The listing builds one solid part. Answer for the finished solid, in the listing's coordinates (mm). Face numbers are marked on the shaded views. A direction names the side the tool comes from. Coordinates: 2 decimals unless noted, no trailing zeros. Write each loop counter-clockwise with the first axis right and the second up, starting at its lowest first coordinate (ties: lowest second). Pieces come first, ordered by that corner, then holes.
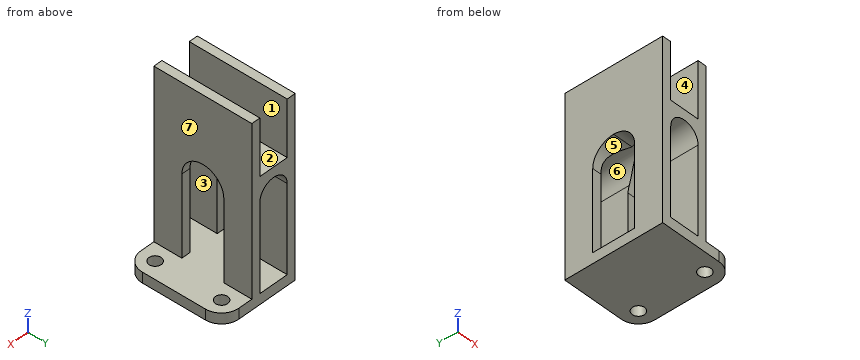
from build123d import *

# Parameters (mm, degrees)
F1_DEPTH     = 28
F2_R         = 1.75
F3_DEPTH     = 25
F4_W         = 12
F4_H         = 29
F5_DEPTH     = 25
F6_T4_DEPTH  = 28
F6_T10_DEPTH = 28
F6_T16_DEPTH = 28
F6_T23_DEPTH = 28
F6_T29_DEPTH = 28
F6_T35_DEPTH = 28
F6_T41_DEPTH = 28
F6_T47_DEPTH = 28
F6_T54_DEPTH = 28
F6_T60_DEPTH = 28
F7_R         = 5.99999
F8_R         = 5


# Not quite as in the source:
# - a fillet or chamfer that OpenCascade refuses, or shapes differently, is made with other operations: its cross-section is extruded or revolved along the edge and cut away or added
# - a fillet or chamfer is up to 0.001 mm smaller than in the source, because OpenCascade refuses the exact size


with BuildPart() as f1:
    # F0 (on Front) → F1 (new body)
    with BuildSketch(Plane.XZ):
        Polygon((-4.25, 25.5), (-6.75, 25.5), (-6.75, -22.5), (-6.75, -25.5), (-4.25, -25.5), (4.25, -25.5), (6.75, -25.5), (15.75, -25.5), (15.75, -22.5), (6.75, -22.5), (6.75, 25.5), (4.25, 25.5), (4.25, 9.5), (0, 9.5), (-4.25, 9.5), align=None)
        Polygon((4.25, -22.5), (-4.25, -22.5), (-4.25, 6.6576944664), (0, 6.6576944664), (4.25, 6.6576944664), align=None, mode=Mode.SUBTRACT)
    extrude(amount=F1_DEPTH)

    # F2 (on face) → F3 (cut)
    with BuildSketch(Plane(origin=(0, 0, -25.5), x_dir=(1, 0, 0), z_dir=(0, 0, -1))):
        with Locations((11.25, 23.5)):
            Circle(F2_R)
        with Locations((11.25, 4.5)):
            Circle(F2_R)
    extrude(amount=-F3_DEPTH, mode=Mode.SUBTRACT)

    # F4 (on face) → F5 (cut)
    with BuildSketch(Plane.YZ.offset(6.75)):
        with Locations((-14, -8)):
            Rectangle(F4_W, F4_H)
    extrude(amount=-F5_DEPTH, mode=Mode.SUBTRACT)

    # F6: fillet of radius 4.25 on 2 edges, made by hand


with BuildPart() as f6_tool2:
    # F6_s3 → F6_t4 (new body)
    with BuildSketch(Plane.XZ):
        with BuildLine():
            ThreePointArc((0, 6.6576944664), (3.00520382, 5.4128982865), (4.25, 2.4076944664))
            Line((4.25, 2.4076944664), (4.25, 6.6576944664))
            Line((4.25, 6.6576944664), (0, 6.6576944664))
        make_face()
    extrude(amount=F6_T4_DEPTH)

    split(bisect_by=Plane.XZ.offset(8), keep=Keep.BOTTOM)

    split(bisect_by=Plane.XY.offset(6.5), keep=Keep.TOP)


with BuildPart() as f1_1:
    add(f1.part)

    # F6_t1: union F6_tool2
    add(f6_tool2.part)


with BuildPart() as f6_tool8:
    # F6_s9 → F6_t10 (new body)
    with BuildSketch(Plane.XZ):
        with BuildLine():
            ThreePointArc((0, 6.6576944664), (3.00520382, 5.4128982865), (4.25, 2.4076944664))
            Line((4.25, 2.4076944664), (4.25, 6.6576944664))
            Line((4.25, 6.6576944664), (0, 6.6576944664))
        make_face()
    extrude(amount=F6_T10_DEPTH)

    split(bisect_by=Plane.XZ.offset(8), keep=Keep.BOTTOM)

    split(bisect_by=Plane.XY.offset(6.5), keep=Keep.BOTTOM)


with BuildPart() as f1_2:
    add(f1_1.part)

    # F6_t7: union F6_tool8
    add(f6_tool8.part)


with BuildPart() as f6_tool14:
    # F6_s15 → F6_t16 (new body)
    with BuildSketch(Plane.XZ):
        with BuildLine():
            ThreePointArc((0, 6.6576944664), (3.00520382, 5.4128982865), (4.25, 2.4076944664))
            Line((4.25, 2.4076944664), (4.25, 6.6576944664))
            Line((4.25, 6.6576944664), (0, 6.6576944664))
        make_face()
    extrude(amount=F6_T16_DEPTH)

    split(bisect_by=Plane.XZ.offset(8), keep=Keep.TOP)

    split(bisect_by=Plane.XY.offset(6.5), keep=Keep.TOP)

    split(bisect_by=Plane.XZ.offset(20), keep=Keep.BOTTOM)


with BuildPart() as f1_3:
    add(f1_2.part)

    # F6_t13: union F6_tool14
    add(f6_tool14.part)


with BuildPart() as f6_tool21:
    # F6_s22 → F6_t23 (new body)
    with BuildSketch(Plane.XZ):
        with BuildLine():
            ThreePointArc((0, 6.6576944664), (3.00520382, 5.4128982865), (4.25, 2.4076944664))
            Line((4.25, 2.4076944664), (4.25, 6.6576944664))
            Line((4.25, 6.6576944664), (0, 6.6576944664))
        make_face()
    extrude(amount=F6_T23_DEPTH)

    split(bisect_by=Plane.XY.offset(6.5), keep=Keep.TOP)

    split(bisect_by=Plane.XZ.offset(20), keep=Keep.TOP)


with BuildPart() as f1_4:
    add(f1_3.part)

    # F6_t20: union F6_tool21
    add(f6_tool21.part)


with BuildPart() as f6_tool27:
    # F6_s28 → F6_t29 (new body)
    with BuildSketch(Plane.XZ):
        with BuildLine():
            ThreePointArc((0, 6.6576944664), (3.00520382, 5.4128982865), (4.25, 2.4076944664))
            Line((4.25, 2.4076944664), (4.25, 6.6576944664))
            Line((4.25, 6.6576944664), (0, 6.6576944664))
        make_face()
    extrude(amount=F6_T29_DEPTH)

    split(bisect_by=Plane.XY.offset(6.5), keep=Keep.BOTTOM)

    split(bisect_by=Plane.XZ.offset(20), keep=Keep.TOP)


with BuildPart() as f1_5:
    add(f1_4.part)

    # F6_t26: union F6_tool27
    add(f6_tool27.part)


with BuildPart() as f6_tool33:
    # F6_s34 → F6_t35 (new body)
    with BuildSketch(Plane.XZ):
        with BuildLine():
            ThreePointArc((-4.25, 2.4076944664), (-3.00520382, 5.4128982865), (0, 6.6576944664))
            Line((0, 6.6576944664), (-4.25, 6.6576944664))
            Line((-4.25, 6.6576944664), (-4.25, 2.4076944664))
        make_face()
    extrude(amount=F6_T35_DEPTH)

    split(bisect_by=Plane.XZ.offset(8), keep=Keep.BOTTOM)

    split(bisect_by=Plane.XY.offset(6.5), keep=Keep.BOTTOM)


with BuildPart() as f1_6:
    add(f1_5.part)

    # F6_t32: union F6_tool33
    add(f6_tool33.part)


with BuildPart() as f6_tool39:
    # F6_s40 → F6_t41 (new body)
    with BuildSketch(Plane.XZ):
        with BuildLine():
            ThreePointArc((-4.25, 2.4076944664), (-3.00520382, 5.4128982865), (0, 6.6576944664))
            Line((0, 6.6576944664), (-4.25, 6.6576944664))
            Line((-4.25, 6.6576944664), (-4.25, 2.4076944664))
        make_face()
    extrude(amount=F6_T41_DEPTH)

    split(bisect_by=Plane.XZ.offset(8), keep=Keep.BOTTOM)

    split(bisect_by=Plane.XY.offset(6.5), keep=Keep.TOP)


with BuildPart() as f1_7:
    add(f1_6.part)

    # F6_t38: union F6_tool39
    add(f6_tool39.part)


with BuildPart() as f6_tool45:
    # F6_s46 → F6_t47 (new body)
    with BuildSketch(Plane.XZ):
        with BuildLine():
            ThreePointArc((-4.25, 2.4076944664), (-3.00520382, 5.4128982865), (0, 6.6576944664))
            Line((0, 6.6576944664), (-4.25, 6.6576944664))
            Line((-4.25, 6.6576944664), (-4.25, 2.4076944664))
        make_face()
    extrude(amount=F6_T47_DEPTH)

    split(bisect_by=Plane.XZ.offset(20), keep=Keep.BOTTOM)

    split(bisect_by=Plane.XZ.offset(8), keep=Keep.TOP)

    split(bisect_by=Plane.XY.offset(6.5), keep=Keep.TOP)


with BuildPart() as f1_8:
    add(f1_7.part)

    # F6_t44: union F6_tool45
    add(f6_tool45.part)


with BuildPart() as f6_tool52:
    # F6_s53 → F6_t54 (new body)
    with BuildSketch(Plane.XZ):
        with BuildLine():
            ThreePointArc((-4.25, 2.4076944664), (-3.00520382, 5.4128982865), (0, 6.6576944664))
            Line((0, 6.6576944664), (-4.25, 6.6576944664))
            Line((-4.25, 6.6576944664), (-4.25, 2.4076944664))
        make_face()
    extrude(amount=F6_T54_DEPTH)

    split(bisect_by=Plane.XZ.offset(20), keep=Keep.TOP)

    split(bisect_by=Plane.XY.offset(6.5), keep=Keep.BOTTOM)


with BuildPart() as f1_9:
    add(f1_8.part)

    # F6_t51: union F6_tool52
    add(f6_tool52.part)


with BuildPart() as f6_tool58:
    # F6_s59 → F6_t60 (new body)
    with BuildSketch(Plane.XZ):
        with BuildLine():
            ThreePointArc((-4.25, 2.4076944664), (-3.00520382, 5.4128982865), (0, 6.6576944664))
            Line((0, 6.6576944664), (-4.25, 6.6576944664))
            Line((-4.25, 6.6576944664), (-4.25, 2.4076944664))
        make_face()
    extrude(amount=F6_T60_DEPTH)

    split(bisect_by=Plane.XZ.offset(20), keep=Keep.TOP)

    split(bisect_by=Plane.XY.offset(6.5), keep=Keep.TOP)


with BuildPart() as f1_10:
    add(f1_9.part)

    # F6_t57: union F6_tool58
    add(f6_tool58.part)

    # F7 (radius 6 in the source; OpenCascade refuses exactly that, so slightly less here)
    f7_edges = [f1_10.edges().sort_by_distance(p)[0] for p in [
        (3.948484, -20, 6.5),
        (-3.948484, -20, 6.5),
        (-3.948484, -8, 6.5),
        (3.948484, -8, 6.5),
    ]]
    fillet(f7_edges, radius=F7_R)

    # F8
    f8_edges = [f1_10.edges().sort_by_distance(p)[0] for p in [
        (15.75, 0, -24),
        (15.75, -28, -24),
    ]]
    fillet(f8_edges, radius=F8_R)


solid = f1_10.part
Q1. Determine the mould class of the marked faces 1, 2 and 3 for opening direction Z: released by +Z, released by -Z, zero draft, split by the parting line, or undercut.
Answers below:
face 1: zero draft
face 2: released by +Z
face 3: undercut
Q2. Which of the six approach directions +Z, -Z, +X, -X, +Y, -Y give full straight-line access (tool end or side, diameter ignored) to the marked faces 4, 5, 6 and 7?
Answers below:
face 4: +Z, +Y, -Y
face 5: +X, -X
face 6: +Y, -Y
face 7: +Z, +X, +Y, -Y
Q3. The part is cut by section B-B, the plane x = 0. Write down the section's boundary in (y, z), then the cut area to 3 significant figures.
Answers below:
outline: (-28, -25.5) - (0, -25.5) - (0, -22.5) - (-28, -22.5) - close; (-28, 6.66) - (0, 6.66) - (0, 9.5) - (-28, 9.5) - close
area: 164 mm2
Q4. Find the intervals of material crossed by probe 1 along X at (y, z) = (-6.75, -21.5); probe 2 along Y at (x, z) = (11.25, -24.15), in increasing order.
Answers below:
probe 1: x = -6.75 to -4.25, 4.25 to 6.75
probe 2: y = -27.97 to -25.25, -21.75 to -6.25, -2.75 to -0.03
Q5. The part is cut by section D-D, the plane y = -11.75. Write down the section's boundary in (x, z), then the cut area to 3 significant figures.
Answers below:
outline: (-6.75, -25.5) - (15.75, -25.5) - (15.75, -22.5) - (-6.75, -22.5) - close; (-6.75, 6.06) - (-2.17, 6.06) arc R4.25 cw to (2.17, 6.06) - (6.75, 6.06) - (6.75, 25.5) - (4.25, 25.5) - (4.25, 9.5) - (-4.25, 9.5) - (-4.25, 25.5) - (-6.75, 25.5) - close
area: 192 mm2
Q6. Given pin 1 (4 mm diameter, centred on y = -3.5, z = -4.5, fed in from +X); pin 2 (11 mm diameter, centred on x = 8, y = -8.5, fed in from +Z); pin 3 (3 mm diameter, centred on x = 11.25, y = -4.5, fed in from +Z); pin 4 (7 mm diameter, centred on x = -0.5, y = -10, fed in from +Z), each flat-ended and moving along its own axis, determine where each tip first touches the part or whether it passes through.
Answers below:
pin 1: stops at x = 6.75
pin 2: stops at z = 25.5
pin 3: passes through
pin 4: stops at z = 9.5
Q7. The part is cut by section C-C, the plane z = -20.5. Write down the section's boundary in (x, y).
Answers below:
outline: (-6.75, -28) - (-4.25, -28) - (-4.25, -20) - (-6.75, -20) - close; (-6.75, -8) - (-4.25, -8) - (-4.25, 0) - (-6.75, 0) - close; (4.25, -28) - (6.75, -28) - (6.75, -20) - (4.25, -20) - close; (4.25, -8) - (6.75, -8) - (6.75, 0) - (4.25, 0) - close
Q8. The part is cut by section A-A, the plane z = 13. Write down the section's boundary in (x, y), then the cut area to 3 significant figures.
Answers below:
outline: (-6.75, -28) - (-4.25, -28) - (-4.25, 0) - (-6.75, 0) - close; (4.25, -28) - (6.75, -28) - (6.75, 0) - (4.25, 0) - close
area: 140 mm2
